Geometry check sheet. Reference: the model listing, model coordinates, mm. A direction names the side the tool comes from. Round coordinates to 2 decimals unless told otherwise and drop trailing zeros. Order: outer loops, then holes, each group sorted by start corner. A loop starts at its lowest first (then second) coordinate and runs counter-clockwise, first axis right, second up. Notation, with made-up numbers: (28.25, -37.5) - (44.25, -37.5) arc R22 ccw to (44.25, -2.5) - close; hole circle Ø11 at (20, 6). An arc over 180 degrees is marked (long way). Write each question's results on one line, items separated by ' | '.
```python
from build123d import *

# Parameters (mm, degrees)
SKETCH1_W           = 181
SKETCH1_H           = 75.57
BOSS_EXTRUDE2_DEPTH = 9
SKETCH6_W           = 1.5
SKETCH6_H           = 10
SKETCH6_R           = 1.85
SKETCH6_R_2         = 1.25
SKETCH6_W_2         = 6.368125956
SKETCH6_H_2         = 20
SKETCH6_W_3         = 6.368125955
SKETCH6_W_4         = 10
SKETCH6_H_3         = 1.5
SKETCH6_R_3         = 1.5
CUT_EXTRUDE7_DEPTH  = 9


with BuildPart() as part:
    # Sketch1 → Boss-Extrude2 (new body)
    with BuildSketch(Plane.XY):
        Rectangle(SKETCH1_W, SKETCH1_H)
    extrude(amount=BOSS_EXTRUDE2_DEPTH)

    # Sketch6 → Cut-Extrude7 (cut)
    with BuildSketch(Plane.XY.offset(9)):
        Polygon((90.5, -25.503407437), (0, -37.785), (90.5, -37.785), align=None)
        Polygon((90.5, 37.785), (0, 37.785), (90.5, 25.503407437), align=None)
        with Locations((87.75, -0.017122468)):
            Rectangle(SKETCH6_W, SKETCH6_H)
        with Locations((83, 0)):
            Circle(SKETCH6_R)
        with Locations((83, -12.753407437)):
            Circle(SKETCH6_R)
        with Locations((70.3, -12.753407437)):
            Circle(SKETCH6_R)
        with Locations((70.3, 0)):
            Circle(SKETCH6_R)
        with Locations((70.3, 12.753407437)):
            Circle(SKETCH6_R)
        with Locations((83, 12.753407437)):
            Circle(SKETCH6_R)
        Polygon((18.699571513, 32.929403247), (28.501771515, 31.599164279), (28.260126082, 29.976752052), (18.476794857, 31.446038639), align=None)
        with Locations((10.504840582, 24)):
            Circle(SKETCH6_R_2)
        with Locations((0.504840582, 24)):
            Circle(SKETCH6_R_2)
        with Locations((-9.454971277, 21.080969171)):
            Rectangle(SKETCH6_W_2, SKETCH6_H_2)
        with Locations((-9.205288194, -21.08)):
            Rectangle(SKETCH6_W_3, SKETCH6_H_2)
        with Locations((0.504840582, -24)):
            Circle(SKETCH6_R_2)
        with Locations((10.504840582, -24)):
            Circle(SKETCH6_R_2)
        Polygon((18.472571869, -32.963494813), (28.501771515, -31.60245013), (28.279412419, -30.118876563), (18.270858535, -31.477119446), align=None)
        with Locations((-28.962631903, 35.035)):
            Rectangle(SKETCH6_W_4, SKETCH6_H_3)
        with Locations((-76.947155779, 35.035)):
            Rectangle(SKETCH6_W_4, SKETCH6_H_3)
        with Locations((-67.23, 30.095)):
            Circle(SKETCH6_R_3)
        with BuildLine():
            Line((-90.5, 37.785), (-90.5, 35.274795088))
            ThreePointArc((-90.5, 35.274795088), (-89.587457665, 37.010103297), (-87.786468161, 37.785))
            Line((-87.786468161, 37.785), (-90.5, 37.785))
        make_face()
        with Locations((-87.75, 18.75)):
            Rectangle(SKETCH6_W, SKETCH6_H)
        with Locations((-87.75, -18.75)):
            Rectangle(SKETCH6_W, SKETCH6_H)
        with BuildLine():
            ThreePointArc((-87.786468161, -37.785), (-89.587457665, -37.010103297), (-90.5, -35.274795088))
            Line((-90.5, -35.274795088), (-90.5, -37.785))
            Line((-90.5, -37.785), (-87.786468161, -37.785))
        make_face()
        with Locations((-76.947155779, -35.035)):
            Rectangle(SKETCH6_W_4, SKETCH6_H_3)
        with Locations((-67.23, -30.095)):
            Circle(SKETCH6_R_3)
        with Locations((-28.962631903, -35.035)):
            Rectangle(SKETCH6_W_4, SKETCH6_H_3)
    extrude(amount=-CUT_EXTRUDE7_DEPTH, mode=Mode.SUBTRACT)


solid = part.part
```
(1) Access from +Z, -Z, +X, -X, +Y, -Y to the whole of each face (thin tool, end or side, straight path). Record for faces 4 (the face through (-9, 31.081, 5)), 5 (the face through (-1, 1, 0)).
Answers follow:
face 4: +Z, -Z | face 5: -Z, +X, -X, +Y, -Y
(2) Depth check by flat-ended pin: pin 1 Ø1 at (x, z) = (50.5, 7) entering from -Y. Enter the tip coordinate at first touch or a pass-through.
Answers follow:
pin 1: y = -31
(3) Section check D-D (x = 83). Record the cut outline in (y, z), then the cut area to 3 significant figures.
Answers follow:
outline: (-26.52, 0) - (-14.6, 0) - (-14.6, 9) - (-26.52, 9) - close; (-10.9, 0) - (-1.85, 0) - (-1.85, 9) - (-10.9, 9) - close; (1.85, 0) - (10.9, 0) - (10.9, 9) - (1.85, 9) - close; (14.6, 0) - (26.52, 0) - (26.52, 9) - (14.6, 9) - close | area: 377 mm²
(4) Section check A-A (x = -8). Record the cut outline in (y, z) (3 decimals), then the cut area to 3 significant figures.
Answers follow:
outline: (-37.785, 0) - (-31.08, 0) - (-31.08, 9) - (-37.785, 9) - close; (-11.08, 0) - (11.081, 0) - (11.081, 9) - (-11.08, 9) - close; (31.081, 0) - (37.785, 0) - (37.785, 9) - (31.081, 9) - close | area: 320 mm²
(5) Section check C-C (y = 0). Record the cut outline in (x, z), then the cut area to 3 significant figures.
Answers follow:
outline: (-90.5, 0) - (68.45, 0) - (68.45, 9) - (-90.5, 9) - close; (72.15, 0) - (81.15, 0) - (81.15, 9) - (72.15, 9) - close; (84.85, 0) - (87, 0) - (87, 9) - (84.85, 9) - close; (88.5, 0) - (90.5, 0) - (90.5, 9) - (88.5, 9) - close | area: 1,550 mm²
(6) Material ranges on line 1 (X direction, y = 12.5, z = 7.75); line 2 (X direction, y = -13, z = 6.5); line 3 (Y direction, x = -8, z = 1.25) (3 decimals), recorded low to high.
Answers follow:
line 1: -90.5 to -12.64, -6.27 to 68.47, 72.13 to 81.17, 84.83 to 90.5 | line 2: -90.5 to -12.39, -6.02 to 68.47, 72.13 to 81.17, 84.83 to 90.5 | line 3: -37.785 to -31.08, -11.08 to 11.081, 31.081 to 37.785
(7) Draft check along Y on faces 1 (the face through (90.5, 0, 4)), 2 (the face through (84.71, -0.71, 4.56)), 3 (the face through (44.62, 31.73, 4.56)). Enter one of: released by +Y, released by -Y, zero draft, split by the parting line, or undercut.
Answers follow:
face 1: zero draft | face 2: undercut | face 3: released by +Y
(8) Section check B-B (y = 17.5). Record the cut outline in (x, z).
Answers follow:
outline: (-90.5, 0) - (-88.5, 0) - (-88.5, 9) - (-90.5, 9) - close; (-87, 0) - (-12.64, 0) - (-12.64, 9) - (-87, 9) - close; (-6.27, 0) - (90.5, 0) - (90.5, 9) - (-6.27, 9) - close
